from build123d import *

# Parameters (mm, degrees)
F0_R     = 3.5
F0_W     = 5
F0_H     = 25
F1_DEPTH = 1
F2_W     = 2
F2_H     = 8
F2_W_2   = 1.9999998777
F2_H_2   = 12
F3_DEPTH = 9.5
F4_W     = 23
F4_H     = 35
F5_DEPTH = 1


with BuildPart() as f1:
    # F0 (on Top) → F1 (new body)
    with BuildSketch(Plane.XY):
        with BuildLine():
            Line((-3.5, 20), (-13.5, 10))
            Line((-13.5, 10), (-13.5, -20))
            Line((-13.5, -20), (-3.5, -20))
            Line((-3.5, -20), (-3.5, -26.2619838908))
            Line((-3.5, -26.2619838908), (-28.879, -26.2619838908))
            ThreePointArc((-28.879, -26.2619838908), (-32.4888159516, -23.8965459278), (-36.7523971724, -24.5658314681))
            ThreePointArc((-36.7523971724, -24.5658314681), (-38.907954465, -25.9032249779), (-40.974404202, -27.3745625074))
            ThreePointArc((-40.974404202, -27.3745625074), (-42.1577536748, -29.7619838908), (-40.974404202, -32.1494052742))
            ThreePointArc((-40.974404202, -32.1494052742), (-38.907954465, -33.6207428037), (-36.7523971724, -34.9581363135))
            ThreePointArc((-36.7523971724, -34.9581363135), (-32.4888159516, -35.6274218538), (-28.879, -33.2619838908))
            Line((-28.879, -33.2619838908), (28.879, -33.2619838908))
            ThreePointArc((28.879, -33.2619838908), (32.4888159516, -35.6274218538), (36.7523971724, -34.9581363135))
            ThreePointArc((36.7523971724, -34.9581363135), (38.907954465, -33.6207428037), (40.974404202, -32.1494052742))
            ThreePointArc((40.974404202, -32.1494052742), (42.1577536748, -29.7619838908), (40.974404202, -27.3745625074))
            ThreePointArc((40.974404202, -27.3745625074), (38.907954465, -25.9032249779), (36.7523971724, -24.5658314681))
            ThreePointArc((36.7523971724, -24.5658314681), (32.4888159516, -23.8965459278), (28.879, -26.2619838908))
            Line((28.879, -26.2619838908), (3.5, -26.2619838908))
            Line((3.5, -26.2619838908), (3.5, -20))
            Line((3.5, -20), (13.5, -20))
            Line((13.5, -20), (13.5, 10))
            Line((13.5, 10), (3.5, 20))
            Line((3.5, 20), (3.5, 26.2619838908))
            Line((3.5, 26.2619838908), (28.879, 26.2619838908))
            ThreePointArc((28.879, 26.2619838908), (32.4888159516, 23.8965459278), (36.7523971724, 24.5658314681))
            ThreePointArc((36.7523971724, 24.5658314681), (38.907954465, 25.9032249779), (40.974404202, 27.3745625074))
            ThreePointArc((40.974404202, 27.3745625074), (42.1577536748, 29.7619838908), (40.974404202, 32.1494052742))
            ThreePointArc((40.974404202, 32.1494052742), (38.907954465, 33.6207428037), (36.7523971724, 34.9581363135))
            ThreePointArc((36.7523971724, 34.9581363135), (32.4888159516, 35.6274218538), (28.879, 33.2619838908))
            Line((28.879, 33.2619838908), (-28.879, 33.2619838908))
            ThreePointArc((-28.879, 33.2619838908), (-32.4888159516, 35.6274218538), (-36.7523971724, 34.9581363135))
            ThreePointArc((-36.7523971724, 34.9581363135), (-38.907954465, 33.6207428037), (-40.974404202, 32.1494052742))
            ThreePointArc((-40.974404202, 32.1494052742), (-42.1577536748, 29.7619838908), (-40.974404202, 27.3745625074))
            ThreePointArc((-40.974404202, 27.3745625074), (-38.907954465, 25.9032249779), (-36.7523971724, 24.5658314681))
            ThreePointArc((-36.7523971724, 24.5658314681), (-32.4888159516, 23.8965459278), (-28.879, 26.2619838908))
            Line((-28.879, 26.2619838908), (-3.5, 26.2619838908))
            Line((-3.5, 26.2619838908), (-3.5, 20))
        make_face()
        with Locations((-33.7523971724, -29.7619838908)):
            Circle(F0_R, mode=Mode.SUBTRACT)
        with Locations((33.7523971724, -29.7619838908)):
            Circle(F0_R, mode=Mode.SUBTRACT)
        with Locations((-4, 0)):
            Rectangle(F0_W, F0_H, mode=Mode.SUBTRACT)
        with Locations((-33.7523971724, 29.7619838908)):
            Circle(F0_R, mode=Mode.SUBTRACT)
        with Locations((4, 0)):
            Rectangle(F0_W, F0_H, mode=Mode.SUBTRACT)
        with Locations((33.7523971724, 29.7619838908)):
            Circle(F0_R, mode=Mode.SUBTRACT)
    extrude(amount=F1_DEPTH)

    # F2 (on Top) → F3 (join)
    with BuildSketch(Plane.XY):
        with Locations((10.5, -9)):
            Rectangle(F2_W, F2_H)
        with Locations((10.5000000611, 3)):
            Rectangle(F2_W_2, F2_H_2)
        with Locations((-10.5000000611, 3)):
            Rectangle(F2_W_2, F2_H_2)
    extrude(amount=-F3_DEPTH)

    # F4 (on face) → F5 (join)
    with BuildSketch(Plane(origin=(0, 0, -9.5), x_dir=(1, 0, 0), z_dir=(0, 0, -1))):
        Rectangle(F4_W, F4_H)
    extrude(amount=F5_DEPTH)


solid = f1.part
Model file for the job. Use its own axes, mm. A direction names the side the tool comes from. Round coordinates to 2 decimals unless told otherwise and drop trailing zeros. Loops run counter-clockwise (first coordinate to the right, second up) from the corner with the lowest first, then second, coordinate; pieces in that order, holes last. Notation, with made-up numbers: (64.25, 43) -> (89.25, 43) arc R5 cw to (89.25, 49) -> close; hole circle Ø2 at (-15.5, -13). An arc over 180 degrees is marked (long way). Answer as CSV lines item,"result". Start each with the question number.
1) Pin check, flat tips, straight feed: P1, Ø1.1, axis at x = 13.5, z = 0.5, coming from the +Y side; P2, Ø5, axis at x = 30.5, z = -1, coming from the -Y side; P3, Ø1.1, axis at x = 3.5, z = 0.5, coming from the -Y side; P4, Ø3, axis at x = -19.5, z = -3, coming from the -Y side. Stop position of each tip, or through.
2) Tool access for faces 1 (the face through (-9.5, 3, -5)), 2 (the face through (10, -13, -5)), 3 (the face through (8.6, 14.9, 0.5)), 4 (the face through (10, -5, -5)): list every direction of +Z, -Z, +X, -X, +Y, -Y with a clear straight run to the whole face (end or side of a thin tool).
3) Mould opens along Z. For faces 5 (the face through (-1, 1, 0)), 6 (the face through (0, 0, -10.5)), 7 (the face through (-11, -3, -5)), 8 (the face through (11.5, 0, -5)) say: +Z half, -Z half, draft (parallel to the pull), parting line (faces both ways), or undercut.
4) Probe line 1 along X through (y, z) = (6.5, -1.5); line 2 along Z through (x, y) = (-22.5, -30); line 3 along Z through (x, y) = (6, -15.5). List the from-to ranges inside material, lowest first.
5) Slice it at A-A (z = -1.25). List the corners of the cut face in (x, y).
6) Slice it at D-D (x = 34). List the corners of the cut face in (y, z).
7) Slice it at B-B (y = 3). List the corners of the cut face in (x, z).
8) Slice it at C-C (x = 25). List the corners of the cut face in (y, z).
Filled in:
1,P1,"stops at y = 33.26"
1,P2,"stops at y = -35.68"
1,P3,"stops at y = -33.26"
1,P4,"passes through"
2,face 1,"+Y, -Y"
2,face 2,"+X, -X, -Y"
2,face 3,"+Z, +X"
2,face 4,"+X, -X"
3,face 5,"undercut"
3,face 6,"-Z half"
3,face 7,"undercut"
3,face 8,"draft"
4,line 1,"x = -11.5 to -9.5, 9.5 to 11.5"
4,line 2,"z = 0 to 1"
4,line 3,"z = -10.5 to -9.5, 0 to 1"
5,outline,"(-11.5, -3) -> (-9.5, -3) -> (-9.5, 9) -> (-11.5, 9) -> close; (9.5, -13) -> (11.5, -13) -> (11.5, -5) -> (9.5, -5) -> close; (9.5, -3) -> (11.5, -3) -> (11.5, 9) -> (9.5, 9) -> close"
6,outline,"(-35.76, 0) -> (-33.25, 0) -> (-33.25, 1) -> (-35.76, 1) -> close; (-26.27, 0) -> (-23.77, 0) -> (-23.77, 1) -> (-26.27, 1) -> close; (23.77, 0) -> (26.27, 0) -> (26.27, 1) -> (23.77, 1) -> close; (33.25, 0) -> (35.76, 0) -> (35.76, 1) -> (33.25, 1) -> close"
7,outline,"(-13.5, 0) -> (-11.5, 0) -> (-11.5, -10.5) -> (11.5, -10.5) -> (11.5, 0) -> (13.5, 0) -> (13.5, 1) -> (6.5, 1) -> (6.5, 0) -> (9.5, 0) -> (9.5, -9.5) -> (-9.5, -9.5) -> (-9.5, 0) -> (-6.5, 0) -> (-6.5, 1) -> (-13.5, 1) -> close; (-1.5, 0) -> (1.5, 0) -> (1.5, 1) -> (-1.5, 1) -> close"
8,outline,"(-33.26, 0) -> (-26.26, 0) -> (-26.26, 1) -> (-33.26, 1) -> close; (26.26, 0) -> (33.26, 0) -> (33.26, 1) -> (26.26, 1) -> close"
